Verification items for this drawing (mm, ordinates from the low corner). A direction names the side the tool comes from. Give positions to 0.01 mm unless a question says otherwise; leave off trailing zeros. Order: outer loops, then holes, each group sorted by start corner. A loop starts at its lowest first (then second) coordinate and runs counter-clockwise, first axis right, second up. Notation, with made-up numbers: M 19,55.25 L 72,55.25 A34 cw 72,87.25 Z; hole C 46,19 d8. An arc over 180 degrees is marked long. Answer as a JSON object with one key per item and string values.
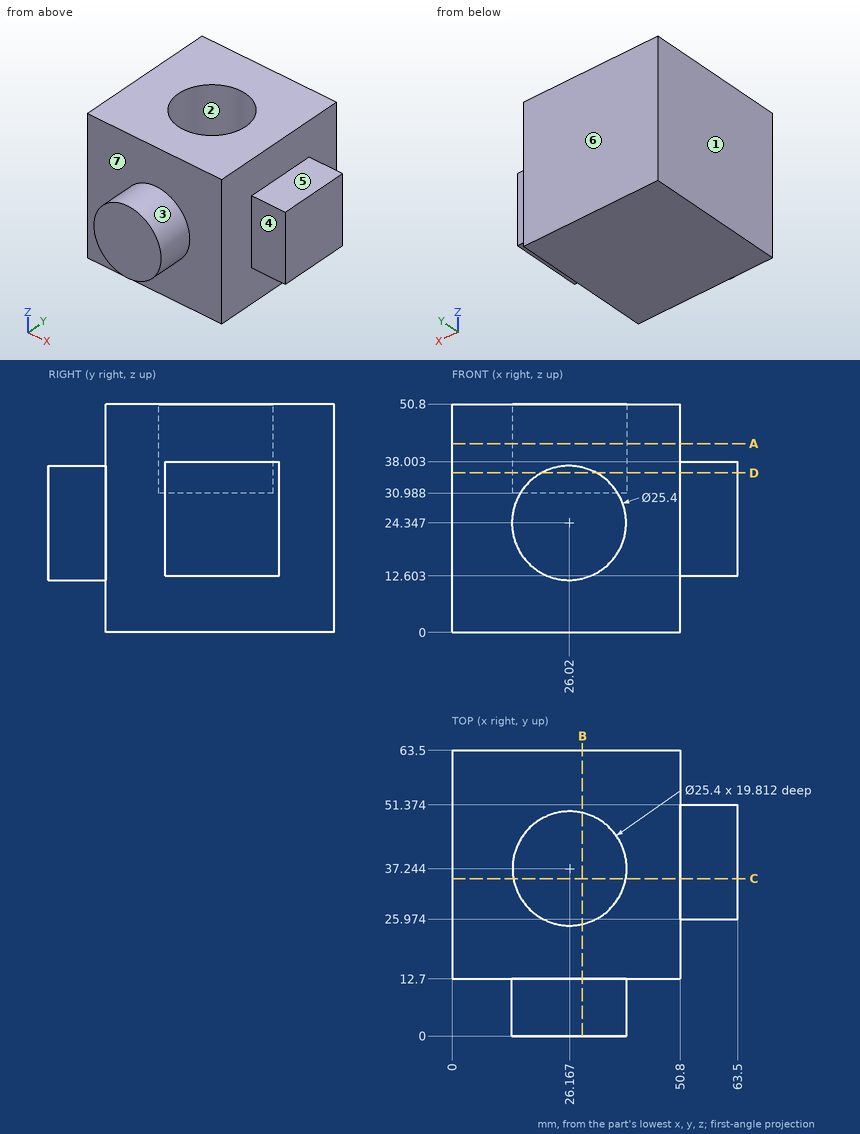
Q1. Section check B-B on x = 29. Record the cut outline in (y, z), then the cut area to 3 significant figures.
Resolved:
{"outline": "M 0,12 L 12.7,12 L 12.7,0 L 63.5,0 L 63.5,50.8 L 49.62,50.8 L 49.62,30.99 L 24.86,30.99 L 24.86,50.8 L 12.7,50.8 L 12.7,36.69 L 0,36.69 Z", "area": "2,400 mm²"}
Q2. Section check A-A on z = 42. Record the cut outline in (x, y), then the cut area to 3 significant figures.
Resolved:
{"outline": "M 0,12.7 L 50.8,12.7 L 50.8,63.5 L 0,63.5 Z; hole C 26.17,37.24 d25.4", "area": "2,070 mm²"}
Q3. Release check for a two-part mould opening along X. For the marked faces 1, 2, 3 and 4 record: +X half, -X half, draft (parallel to the pull), parting line (faces both ways), or undercut.
Resolved:
{"face 1": "-X half", "face 2": "undercut", "face 3": "parting line", "face 4": "draft"}
Q4. Material ranges on L1, parallel to Z at x = 23, y = 40.5; L2, parallel to X at y = 45.5, z = 5; L3, parallel to Y at x = 16.5, z = 43.5 (1 decimal), recorded low to high.
Resolved:
{"L1": "z = 0 to 30.99", "L2": "x = 0 to 50.8", "L3": "y = 12.7 to 29, 45.5 to 63.5"}
Q5. Section check D-D on z = 35.5. Record the cut outline in (x, y) (1 decimal).
Resolved:
{"outline": "M 0,12.7 L 19.9,12.7 L 19.9,0 L 32.1,0 L 32.1,12.7 L 50.8,12.7 L 50.8,26 L 63.5,26 L 63.5,51.4 L 50.8,51.4 L 50.8,63.5 L 0,63.5 Z; hole C 26.2,37.2 d25.4"}
Q6. Section check C-C on y = 35. Record the cut outline in (x, z), then the cut area to 3 significant figures.
Resolved:
{"outline": "M 0,0 L 50.8,0 L 50.8,12.6 L 63.5,12.6 L 63.5,38 L 50.8,38 L 50.8,50.8 L 38.67,50.8 L 38.67,30.99 L 13.67,30.99 L 13.67,50.8 L 0,50.8 Z", "area": "2,410 mm²"}
Q7. Tool access check on the marked faces 5, 6 and 7. Record the directions out of +Z, -Z, +X, -X, +Y, -Y that give a thin tool (end or side, any length) a straight path to the whole face; none if there is none.
Resolved:
{"face 5": "+Z, +X, +Y, -Y", "face 6": "+Z, -Z, +X, -X, +Y", "face 7": "-Y"}
Q8. Gauge pin test, flat ends, axial feed: pin 1 Ø3 at (y, z) = (12.5, 14) entering from +X; pin 2 Ø4 at (y, z) = (16.5, 36.5) entering from -X; pin 3 Ø6.5 at (x, y) = (55, 38.5) entering from +Z; pin 4 Ø4 at (x, z) = (55.5, 11) entering from +Y. Record the tip position at first contact, or that the pin passes through.
Resolved:
{"pin 1": "stops at x = 50.8", "pin 2": "stops at x = 0", "pin 3": "stops at z = 38", "pin 4": "stops at y = 51.37"}
